```python
from build123d import *

# Parameters (mm, degrees)
F0_W     = 22
F0_H     = 3
F1_DEPTH = 100
F3_DEPTH = 4
F4_W     = 4
F4_H     = 3
F4_W_2   = 22
F5_DEPTH = 4
F6_R     = 2.5
F7_DEPTH = 25


with BuildPart() as f1:
    # F0 (on Top) → F1 (new body)
    with BuildSketch(Plane.XY):
        with Locations((11, -1.5)):
            Rectangle(F0_W, F0_H)
    extrude(amount=F1_DEPTH)

    # F2 (on face) → F3 (join)
    with BuildSketch(Plane(origin=(0, 0, 0), x_dir=(1, 0, 0), z_dir=(0, 0, -1))):
        with BuildLine():
            ThreePointArc((4, 0), (5.06066, 0.43934), (5.5, 1.5))
            ThreePointArc((5.5, 1.5), (5.06066, 2.56066), (4, 3))
            ThreePointArc((4, 3), (2.5, 1.5), (4, 0))
        make_face()
        with BuildLine():
            ThreePointArc((19.5, 1.5), (19.06066, 2.56066), (18, 3))
            ThreePointArc((18, 3), (16.5, 1.5), (18, 0))
            ThreePointArc((18, 0), (19.06066, 0.43934), (19.5, 1.5))
        make_face()
    extrude(amount=F3_DEPTH)

    # F4 (on face) → F5 (join)
    with BuildSketch(Plane.XY.offset(100)):
        with Locations((-2, -1.5)):
            Rectangle(F4_W, F4_H)
        with Locations((24, -1.5)):
            Rectangle(F4_W, F4_H)
        with Locations((11, -1.5)):
            Rectangle(F4_W_2, F4_H)
    extrude(amount=-F5_DEPTH)

    # F6 (on face) → F7 (cut)
    with BuildSketch(Plane.XZ.offset(3)):
        with Locations((5, 8)):
            Circle(F6_R)
        with Locations((11, 8)):
            Circle(F6_R)
        with Locations((17, 8)):
            Circle(F6_R)
        with Locations((5, 16)):
            Circle(F6_R)
        with Locations((11, 16)):
            Circle(F6_R)
        with Locations((17, 16)):
            Circle(F6_R)
        with Locations((5, 24)):
            Circle(F6_R)
        with Locations((11, 24)):
            Circle(F6_R)
        with Locations((17, 24)):
            Circle(F6_R)
        with Locations((5, 32)):
            Circle(F6_R)
        with Locations((11, 32)):
            Circle(F6_R)
        with Locations((17, 32)):
            Circle(F6_R)
        with Locations((5, 40)):
            Circle(F6_R)
        with Locations((11, 40)):
            Circle(F6_R)
        with Locations((17, 40)):
            Circle(F6_R)
        with Locations((5, 48)):
            Circle(F6_R)
        with Locations((11, 48)):
            Circle(F6_R)
        with Locations((17, 48)):
            Circle(F6_R)
        with Locations((5, 56)):
            Circle(F6_R)
        with Locations((11, 56)):
            Circle(F6_R)
        with Locations((17, 56)):
            Circle(F6_R)
        with Locations((5, 64)):
            Circle(F6_R)
        with Locations((11, 64)):
            Circle(F6_R)
        with Locations((17, 64)):
            Circle(F6_R)
        with Locations((5, 72)):
            Circle(F6_R)
        with Locations((11, 72)):
            Circle(F6_R)
        with Locations((17, 72)):
            Circle(F6_R)
        with Locations((5, 80)):
            Circle(F6_R)
        with Locations((11, 80)):
            Circle(F6_R)
        with Locations((17, 80)):
            Circle(F6_R)
        with Locations((5, 88)):
            Circle(F6_R)
        with Locations((11, 88)):
            Circle(F6_R)
        with Locations((17, 88)):
            Circle(F6_R)
    extrude(amount=-F7_DEPTH, mode=Mode.SUBTRACT)


solid = f1.part
```
Check sheet for the modelled part. Datum: model origin and axes. Units: mm. A direction names the side the tool comes from. Coordinates: 2 decimals unless noted, no trailing zeros. Write each loop counter-clockwise with the first axis right and the second up, starting at its lowest first coordinate (ties: lowest second). Pieces come first, ordered by that corner, then holes. Notation, with made-up numbers: (72, 18) - (124, 18) arc R11 ccw to (124, 36) - close; hole circle Ø6 at (43.25, -24). An arc over 180 degrees is marked (long way). One line per question, with ' | ' between items.
Item 1: Gauge pin test, flat end, axial feed: P1, Ø1.5, axis at x = 9.5, y = -1, coming from the -Z side. Record the tip position at first contact, or that the pin passes through.
Determined:
P1: stops at z = 0
Item 2: Sectioned sample at A-A on z = 24. Record the boundary of the cut face in (x, y), plus the area to 3 significant figures.
Determined:
outline: (0, -3) - (2.5, -3) - (2.5, 0) - (0, 0) - close; (7.5, -3) - (8.5, -3) - (8.5, 0) - (7.5, 0) - close; (13.5, -3) - (14.5, -3) - (14.5, 0) - (13.5, 0) - close; (19.5, -3) - (22, -3) - (22, 0) - (19.5, 0) - close | area: 21.0 mm2
Item 3: Mould release check, pull along X, two halves, no side actions. Record for faces 4 (the face through (16.67, -1.52, 90.48)), 5 (the face through (0, -2, 47)), 6 (the face through (2, -1, 0)): pulls with the +X half, pulls with the -X half, needs draft (parallel to the pull), parting line crosses it, or undercut.
Determined:
face 4: undercut | face 5: pulls with the -X half | face 6: needs draft
Item 4: Sectioned sample at C-C on z = 46.5. Record the boundary of the cut face in (x, y), plus the area to 3 significant figures.
Determined:
outline: (0, -3) - (3, -3) - (3, 0) - (0, 0) - close; (7, -3) - (9, -3) - (9, 0) - (7, 0) - close; (13, -3) - (15, -3) - (15, 0) - (13, 0) - close; (19, -3) - (22, -3) - (22, 0) - (19, 0) - close | area: 30.0 mm2
Item 5: Sectioned sample at D-D on x = 23. Record the boundary of the cut face in (y, z), plus the area to 3 significant figures.
Determined:
outline: (-3, 96) - (0, 96) - (0, 100) - (-3, 100) - close | area: 12.0 mm2
Item 6: Sectioned sample at B-B on x = 11. Give the number of separate pieces and of enclosed holes in the cut face, plus the area to 3 significant figures.
Determined:
separate pieces: 12 | enclosed holes: 0 | area: 135 mm2
Item 7: Access from +Z, -Z, +X, -X, +Y, -Y to the whole of each face (thin tool, end or side, straight path). Record for faces 1 (the face through (-2, -1, 96)), 2 (the face through (24, -1, 96)), 3 (the face through (6.34, -1.52, 34.11)).
Determined:
face 1: -Z, -X, +Y, -Y | face 2: -Z, +X, +Y, -Y | face 3: +Y, -Y
Item 8: Thickness scan on line 1 (X direction, y = -2.2, z = 33); line 2 (X direction, y = -2.1, z = 22); line 3 (X direction, y = -2.4, z = 76). Record the ranges inside material, lowest first. Write a range as [from, to].
Determined:
line 1: x = [0, 2.71], [7.29, 8.71], [13.29, 14.71], [19.29, 22] | line 2: x = [0, 3.5], [6.5, 9.5], [12.5, 15.5], [18.5, 22] | line 3: x = [0, 22]
